```python
from build123d import *

# Parameters (mm, degrees)
SKETCH_1_R           = 250
EXTRUDE_1_DEPTH      = 3
CUT_EXTRUDE_1_DEPTH  = 4
CUT_EXTRUDE_2_DEPTH  = 4
FILLET_1_R           = 5
FILLET_2_R           = 5
FILLET_3_R           = 5
FILLET_4_R           = 5
FILLET_5_R           = 5
FILLET_6_R           = 5
FILLET_7_R           = 5
FILLET_8_R           = 5
SKETCH_18_R          = 1.5
CUT_EXTRUDE_10_DEPTH = 4
SKETCH_19_R          = 1.5
CUT_EXTRUDE_11_DEPTH = 3
SKETCH_20_R          = 1.6
CUT_EXTRUDE_12_DEPTH = 4
SKETCH_24_R          = 1.5
CUT_EXTRUDE_14_DEPTH = 4
SKETCH_25_R          = 1.5
CUT_EXTRUDE_15_DEPTH = 4
SKETCH_21_R          = 1.5
CUT_EXTRUDE_16_DEPTH = 4
SKETCH_26_R          = 1.6
CUT_EXTRUDE_17_DEPTH = 4
SKETCH_27_R          = 1.5
CUT_EXTRUDE_18_DEPTH = 4
SKETCH_28_R          = 1.5
CUT_EXTRUDE_19_DEPTH = 4
SKETCH_29_W          = 40
SKETCH_29_H          = 40
CUT_EXTRUDE_20_DEPTH = 4
SKETCH_30_R          = 1.5
CUT_EXTRUDE_21_DEPTH = 4
SKETCH_31_R          = 1.5
CUT_EXTRUDE_22_DEPTH = 4
SKETCH_32_R          = 1.5
CUT_EXTRUDE_23_DEPTH = 4


with BuildPart() as part:
    # ｽｹｯﾁ1 → ﾎﾞｽ - 押し出し1 (new body)
    with BuildSketch(Plane.XY):
        Circle(SKETCH_1_R)
    extrude(amount=-EXTRUDE_1_DEPTH)

    # ｽｹｯﾁ2 → ｶｯﾄ - 押し出し1 (cut, through all)
    with BuildSketch(Plane.XY):
        Polygon((0, 190), (70, 190), (70, 250), (0, 250), (-70, 250), (-70, 190), align=None)
    extrude(amount=-CUT_EXTRUDE_1_DEPTH, mode=Mode.SUBTRACT)

    # ｽｹｯﾁ3 → ｶｯﾄ - 押し出し2 (cut, through all)
    with BuildSketch(Plane.XY):
        Polygon((0, -250), (70, -250), (70, -190), (0, -190), (-70, -190), (-70, -250), align=None)
    extrude(amount=-CUT_EXTRUDE_2_DEPTH, mode=Mode.SUBTRACT)

    # ﾌｨﾚｯﾄ1
    fillet_1_edges = [part.edges().sort_by_distance(p)[0] for p in [
        (-70, 240, -1.5),
    ]]
    fillet(fillet_1_edges, radius=FILLET_1_R)

    # ﾌｨﾚｯﾄ2
    fillet_2_edges = [part.edges().sort_by_distance(p)[0] for p in [
        (70, 240, -1.5),
    ]]
    fillet(fillet_2_edges, radius=FILLET_2_R)

    # ﾌｨﾚｯﾄ3
    fillet_3_edges = [part.edges().sort_by_distance(p)[0] for p in [
        (70, 190, -1.5),
    ]]
    fillet(fillet_3_edges, radius=FILLET_3_R)

    # ﾌｨﾚｯﾄ4
    fillet_4_edges = [part.edges().sort_by_distance(p)[0] for p in [
        (-70, 190, -1.5),
    ]]
    fillet(fillet_4_edges, radius=FILLET_4_R)

    # ﾌｨﾚｯﾄ5
    fillet_5_edges = [part.edges().sort_by_distance(p)[0] for p in [
        (-70, -240, -1.5),
    ]]
    fillet(fillet_5_edges, radius=FILLET_5_R)

    # ﾌｨﾚｯﾄ6
    fillet_6_edges = [part.edges().sort_by_distance(p)[0] for p in [
        (70, -190, -1.5),
    ]]
    fillet(fillet_6_edges, radius=FILLET_6_R)

    # ﾌｨﾚｯﾄ7
    fillet_7_edges = [part.edges().sort_by_distance(p)[0] for p in [
        (70, -240, -1.5),
    ]]
    fillet(fillet_7_edges, radius=FILLET_7_R)

    # ﾌｨﾚｯﾄ8
    fillet_8_edges = [part.edges().sort_by_distance(p)[0] for p in [
        (-70, -190, -1.5),
    ]]
    fillet(fillet_8_edges, radius=FILLET_8_R)

    # ｽｹｯﾁ18 → ｶｯﾄ - 押し出し10 (cut, through all)
    with BuildSketch(Plane.XY):
        with Locations((-100, 144.75)):
            Circle(SKETCH_18_R)
        with Locations((-100, 115.25)):
            Circle(SKETCH_18_R)
        with Locations((-100, -115.25)):
            Circle(SKETCH_18_R)
        with Locations((-100, -144.75)):
            Circle(SKETCH_18_R)
    extrude(amount=-CUT_EXTRUDE_10_DEPTH, mode=Mode.SUBTRACT)

    # ｽｹｯﾁ19 → ｶｯﾄ - 押し出し11 (cut)
    with BuildSketch(Plane.XY):
        with Locations((-160, 10.5)):
            Circle(SKETCH_19_R)
        with Locations((-160, -10.5)):
            Circle(SKETCH_19_R)
    extrude(amount=-CUT_EXTRUDE_11_DEPTH, mode=Mode.SUBTRACT)

    # ｽｹｯﾁ20 → ｶｯﾄ - 押し出し12 (cut, through all)
    with BuildSketch(Plane.XY):
        with Locations((-243, 7.75)):
            Circle(SKETCH_20_R)
        with Locations((-243, -7.75)):
            Circle(SKETCH_20_R)
        with Locations((-163.855062784, 179.612307206)):
            Circle(SKETCH_20_R)
        with Locations((-174.967177203, 168.806248112)):
            Circle(SKETCH_20_R)
        with Locations((-163.855062784, -179.612307206)):
            Circle(SKETCH_20_R)
        with Locations((-174.967177203, -168.806248112)):
            Circle(SKETCH_20_R)
    extrude(amount=-CUT_EXTRUDE_12_DEPTH, mode=Mode.SUBTRACT)

    # ｽｹｯﾁ24 → ｶｯﾄ - 押し出し14 (cut, through all)
    with BuildSketch(Plane.XY):
        with Locations((225, 10)):
            Circle(SKETCH_24_R)
        with Locations((225, -10)):
            Circle(SKETCH_24_R)
        with Locations((210, -10)):
            Circle(SKETCH_24_R)
        with Locations((210, 10)):
            Circle(SKETCH_24_R)
    extrude(amount=-CUT_EXTRUDE_14_DEPTH, mode=Mode.SUBTRACT)

    # ｽｹｯﾁ25 → ｶｯﾄ - 押し出し15 (cut, through all)
    with BuildSketch(Plane.XY):
        with Locations((-225, 10)):
            Circle(SKETCH_25_R)
        with Locations((-225, -10)):
            Circle(SKETCH_25_R)
        with Locations((-210, -10)):
            Circle(SKETCH_25_R)
        with Locations((-210, 10)):
            Circle(SKETCH_25_R)
    extrude(amount=-CUT_EXTRUDE_15_DEPTH, mode=Mode.SUBTRACT)

    # ｽｹｯﾁ21 → ｶｯﾄ - 押し出し16 (cut, through all)
    with BuildSketch(Plane.XY):
        with Locations((137.80005554, 158.464963614)):
            Circle(SKETCH_21_R)
        with Locations((137.80005554, -158.464963614)):
            Circle(SKETCH_21_R)
        with Locations((-137.80005554, -158.464963614)):
            Circle(SKETCH_21_R)
        with Locations((-137.80005554, 158.464963614)):
            Circle(SKETCH_21_R)
    extrude(amount=-CUT_EXTRUDE_16_DEPTH, mode=Mode.SUBTRACT)

    # ｽｹｯﾁ26 → ｶｯﾄ - 押し出し17 (cut, through all)
    with BuildSketch(Plane.XY):
        with Locations((174.967177203, -168.806248112)):
            Circle(SKETCH_26_R)
        with Locations((163.855062784, -179.612307206)):
            Circle(SKETCH_26_R)
        with Locations((243, -7.75)):
            Circle(SKETCH_26_R)
        with Locations((243, 7.75)):
            Circle(SKETCH_26_R)
        with Locations((174.967177203, 168.806248112)):
            Circle(SKETCH_26_R)
        with Locations((163.855062784, 179.612307206)):
            Circle(SKETCH_26_R)
    extrude(amount=-CUT_EXTRUDE_17_DEPTH, mode=Mode.SUBTRACT)

    # ｽｹｯﾁ27 → ｶｯﾄ - 押し出し18 (cut, through all)
    with BuildSketch(Plane.XY):
        with Locations((-10, 180)):
            Circle(SKETCH_27_R)
        with Locations((10, 180)):
            Circle(SKETCH_27_R)
        with Locations((10, 165)):
            Circle(SKETCH_27_R)
        with Locations((-10, 165)):
            Circle(SKETCH_27_R)
        with Locations((10, -180)):
            Circle(SKETCH_27_R)
        with Locations((10, -165)):
            Circle(SKETCH_27_R)
        with Locations((-10, -165)):
            Circle(SKETCH_27_R)
        with Locations((-10, -180)):
            Circle(SKETCH_27_R)
    extrude(amount=-CUT_EXTRUDE_18_DEPTH, mode=Mode.SUBTRACT)

    # ｽｹｯﾁ28 → ｶｯﾄ - 押し出し19 (cut, through all)
    with BuildSketch(Plane.XY):
        with Locations((17.5, 130)):
            Circle(SKETCH_28_R)
        with Locations((82.5, 120)):
            Circle(SKETCH_28_R)
        with Locations((17.5, 50)):
            Circle(SKETCH_28_R)
        with Locations((82.5, 50)):
            Circle(SKETCH_28_R)
        with Locations((17.5, -50)):
            Circle(SKETCH_28_R)
        with Locations((82.5, -60)):
            Circle(SKETCH_28_R)
        with Locations((17.5, -130)):
            Circle(SKETCH_28_R)
        with Locations((82.5, -130)):
            Circle(SKETCH_28_R)
        Polygon((10, 40), (90, 40), (90, 0), (90, -40), (10, -40), (10, 1.027968607), align=None)
    extrude(amount=-CUT_EXTRUDE_19_DEPTH, mode=Mode.SUBTRACT)

    # ｽｹｯﾁ29 → ｶｯﾄ - 押し出し20 (cut, through all)
    with BuildSketch(Plane.XY):
        with Locations((-25, -130)):
            Rectangle(SKETCH_29_W, SKETCH_29_H)
        with Locations((-25, 130)):
            Rectangle(SKETCH_29_W, SKETCH_29_H)
    extrude(amount=-CUT_EXTRUDE_20_DEPTH, mode=Mode.SUBTRACT)

    # ｽｹｯﾁ30 → ｶｯﾄ - 押し出し21 (cut, through all)
    with BuildSketch(Plane.XY):
        with Locations((110, 43.5)):
            Circle(SKETCH_30_R)
        with Locations((174, 43.5)):
            Circle(SKETCH_30_R)
        with Locations((110, -43.5)):
            Circle(SKETCH_30_R)
        with Locations((174, -43.5)):
            Circle(SKETCH_30_R)
    extrude(amount=-CUT_EXTRUDE_21_DEPTH, mode=Mode.SUBTRACT)

    # ｽｹｯﾁ31 → ｶｯﾄ - 押し出し22 (cut, through all)
    with BuildSketch(Plane.XY):
        with Locations((-20, 70)):
            Circle(SKETCH_31_R)
        with Locations((-110, 70)):
            Circle(SKETCH_31_R)
        with Locations((-110, -70)):
            Circle(SKETCH_31_R)
        with Locations((-17.141016151, -70)):
            Circle(SKETCH_31_R)
    extrude(amount=-CUT_EXTRUDE_22_DEPTH, mode=Mode.SUBTRACT)

    # ｽｹｯﾁ32 → ｶｯﾄ - 押し出し23 (cut, through all)
    with BuildSketch(Plane.XY):
        with Locations((-120, 95)):
            Circle(SKETCH_32_R)
        with Locations((-120, -95)):
            Circle(SKETCH_32_R)
        with Locations((70, 145)):
            Circle(SKETCH_32_R)
        with Locations((70, -145)):
            Circle(SKETCH_32_R)
    extrude(amount=-CUT_EXTRUDE_23_DEPTH, mode=Mode.SUBTRACT)


solid = part.part
```
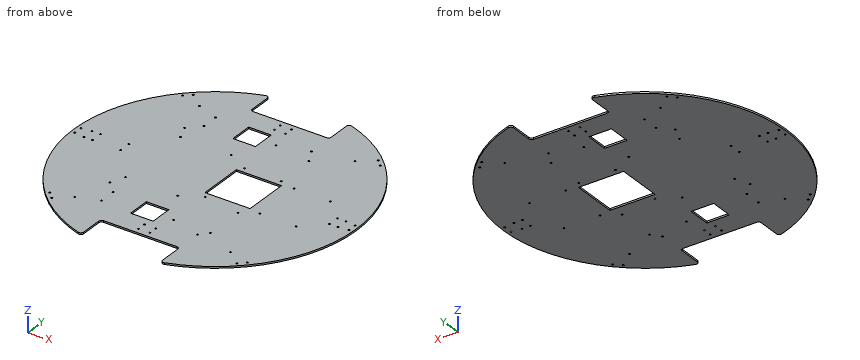
Geometry: final body of the model. Coordinates: model frame, mm. Coordinates: 2 decimals unless noted, no trailing zeros. Write each loop counter-clockwise with the first axis right and the second up, starting at its lowest first coordinate (ties: lowest second). Pieces come first, ordered by that corner, then holes. Notation, with made-up numbers: M -7,37.25 L 10,37.25 A27 ccw 10,63.25 Z; hole C 65.25,12 d2. An arc over 180 degrees is marked long. Answer as CSV lines item,"result". Start each with the question number.
Q1. Cut plane B-B on y = -206.5. Return the cut outline in (x, z), then the cut area to 3 significant figures.
Q2. Cut plane A-A on x = 43.5. Return the cut outline in (y, z), then the cut area to 3 significant figures.
Q3. Cut plane C-C on z = -0.7. Count the separate pieces of the cut face and the enclosed holes in it, then the cut area to 3 significant figures.
Q4. Pin query (flat end, axial travel): P1, Ø2.5, axis at x = -160, y = 10.5, coming from the -Z side; P2, Ø1.5, axis at x = 174, z = -0.5, coming from the +Y side. Return the tip coordinate at first contact, or that it passes through.
Q5. Cut plane D-D on x = 202.5. Return the cut outline in (y, z).
Q6. Line query: line 1 (Y direction, x = -34, z = -0.3); line 2 (X direction, y = 8, z = -0.65); line 3 (Y direction, x = 17.5, z = -1.3). Output: solid intervals per line, ascending. Write a range as from..to.
Findings below:
1,outline,"M -140.92,-3 L -70,-3 L -70,0 L -140.92,0 Z; M 70,-3 L 140.92,-3 L 140.92,0 L 70,0 Z"
1,area,"426 mm2"
2,outline,"M -190,-3 L -40,-3 L -40,0 L -190,0 Z; M 40,-3 L 190,-3 L 190,0 L 40,0 Z"
2,area,"900 mm2"
3,separate pieces,"1"
3,enclosed holes,"61"
3,area,"170,000 mm2"
4,P1,"passes through"
4,P2,"stops at y = 180.23"
5,outline,"M -146.61,-3 L 146.61,-3 L 146.61,0 L -146.61,0 Z"
6,line 1,"y = -190..-150, -110..110, 150..190"
6,line 2,"x = -249.87..-244.58, -241.42..10, 90..241.42, 244.58..249.87"
6,line 3,"y = -190..-131.5, -128.5..-51.5, -48.5..-40, 40..48.5, 51.5..128.5, 131.5..190"
